Design review of the part built by this model. Coordinates are the model's own, in mm. A direction names the side the tool comes from. Round coordinates to 2 decimals unless told otherwise and drop trailing zeros. Order: outer loops, then holes, each group sorted by start corner. A loop starts at its lowest first (then second) coordinate and runs counter-clockwise, first axis right, second up.
Autodesk Inventor part; units mm, degrees
ref_plane "YZ Plane" through (0, 0, 0) normal (1, 0, 0) x (0, 1, 0)
ref_plane "XZ Plane" through (0, 0, 0) normal (0, 1, 0) x (-1, 0, 0)
ref_plane "XY Plane" through (0, 0, 0) normal (0, 0, 1) x (1, 0, 0)
ref_plane "작업 평면1" through (-380, -430.4083, 1686.95) normal (1, 0, 0) x (0, 1, 0)
sketch "스케치1" plane through (-380, -430.4083, 1686.95) normal (1, 0, 0) x (0, 1, 0)
  circle A0 centre (0, 0) radius 290
  point P0 (430.4083, -1686.95)
  dimension "d0" = 580
extrude "돌출1" add sketch "스케치1" along normal blind 100
sketch "스케치2" plane through (-380, -430.4083, 1686.95) normal (-1, 0, 0) x (0, 0, 1)
  circle A0 centre (0, 0) radius 20
  point P0 (-1686.95, 430.4083)
  dimension "d3" = 40
extrude "돌출2" add sketch "스케치2" along normal blind 10
sketch "스케치3" plane through (-280, -430.4083, 1686.95) normal (1, 0, 0) x (0, 0, -1)
  circle A0 centre (0, 0) radius 225
  circle A1 centre (0, 0) radius 20
  circle A2 centre (0, 0) radius 50
  arc A3 (225, 0) -> (50, 0) centre (137.5, -121.8349) ccw
  arc A4 (0, -225) -> (0, -50) centre (-121.8349, -137.5) ccw
  line L0 (0, 0) -> (159.099, -159.099)
  line L1 (0, 0) -> (225, 0) construction
  line L2 (159.099, -159.099) -> (-159.099, 159.099)
  line L3 (0, 0) -> (159.099, 159.099)
  line L4 (0, 0) -> (225, 0) construction
  line L5 (159.099, 159.099) -> (-159.099, -159.099)
  arc A5 (-159.099, -159.099) -> (-35.3553, -35.3553) centre (-183.3775, -11.0769) ccw
  arc A6 (159.099, 159.099) -> (35.3553, 35.3553) centre (183.3775, 11.0769) ccw
  arc A7 (159.099, -159.099) -> (35.3553, -35.3553) centre (11.0769, -183.3775) ccw
  arc A8 (-225, 0) -> (-50, 0) centre (-137.5, 121.8349) ccw
  arc A9 (-159.099, 159.099) -> (-35.3553, 35.3553) centre (-11.0769, 183.3775) ccw
  arc A10 (0, 225) -> (0, 50) centre (121.8349, 137.5) ccw
  point P0 (1686.95, 430.4083)
  dimension "d6" = 450
  dimension "d7" = 100
  dimension "d10" = 150
  dimension "d11" = 150
  dimension "d12" = 45
  dimension "d13" = 45
  dimension "d14" = 150
  dimension "d16" = 150
  dimension "d17" = 150
  dimension "d18" = 150
  dimension "d19" = 150
  dimension "d20" = 150
extrude "돌출3" cut sketch "스케치3" against normal blind 100 contours A0 A7 A2 A3 | A6 A2 A10 A0 | A0 A5 A2 A4 | A9 A2 A8 A0
fillet "모깎기1" radius 121.75 4 edges at (-330, -380.4083, 1686.95) (-330, -430.4083, 1736.95) (-330, -480.4083, 1686.95) (-330, -430.4083, 1636.95)
fillet "모깎기2" radius 36.25 4 edges at (-330, -205.4083, 1686.95) (-330, -430.4083, 1911.95) (-330, -430.4083, 1461.95) (-330, -655.4083, 1686.95)
properties part number "바퀴"
1) Clearance check with flat-ended pins moving along their axes: P1, Ø1, axis at x = -328.5, y = -226, coming from the +Z side; P2, Ø1, axis at x = -330.5, z = 1648.5, coming from the -Y side; P3, Ø10, axis at x = -313.5, z = 1600.5, coming from the -Y side. State where each tip first meets the part, or that it passes through.
Results:
P1: stops at z = 1893.16
P2: stops at y = -717.91
P3: stops at y = -708.74
2) Take a section at D-D on z = 1927. Give the boundary of the cut face in (x, y).
Results:
outline: (-380, -593.12) - (-280, -593.12) - (-280, -267.69) - (-380, -267.69) - close
3) The part is to be moulded in two halves that separate along X. For faces 1 (the face through (-329.3, -617.76, 1667.31)), 2 (the face through (-390, -430, 1687)), 3 (the face through (-280, -434, 1691)), say which applies: released by +X, released by -X, zero draft, split by the parting line, or undercut.
Results:
face 1: zero draft
face 2: released by -X
face 3: released by +X
4) Take a section at B-B on z = 1621. State how many separate pieces and enclosed holes the cut face has, plus the area to 3 significant figures.
Results:
separate pieces: 3
enclosed holes: 0
area: 41,100 mm2
5) For faces 4 (the face through (-384.93, -431.29, 1666.97)), 5 (the face through (-329.3, -450.049, 1874.297)), list the 3-axis set-ups (+Z, -Z, +X, -X, +Y, -Y) from which the entire face can be reached by the end or side of a thin tool; tool diameter is ignored.
Results:
face 4: -X
face 5: +X, -X
6) To check wall thickness, follow line 1 along Z through (x, y) = (-326, -315.5); line 2 along Y through (x, z) = (-343, 1543); line 3 along Y through (x, z) = (-365, 1758.5). State the ranges of each line that lie inside material, in increasing order.
Results:
line 1: z = 1420.69 to 1611.83, 1711.03 to 1831.49, 1880.4 to 1953.21
line 2: y = -682.16 to -544.18, -402.91 to -274.61, -257.48 to -178.66
line 3: y = -711.44 to -643.73, -541.46 to -434.32, -384.3 to -149.37
7) Take a section at A-A on y = -235. Give the boundary of the cut face in (x, z), plus the area to 3 significant figures.
Results:
outline: (-380, 1472.67) - (-280, 1472.67) - (-280, 1575.41) - (-380, 1575.41) - close; (-380, 1703.49) - (-280, 1703.49) - (-280, 1901.23) - (-380, 1901.23) - close
area: 30,000 mm2
